The listing builds one solid part. Answer for the finished solid, in the listing's coordinates (mm). A direction names the side the tool comes from. Coordinates: 2 decimals unless noted, no trailing zeros. Order: outer loops, then holes, each group sorted by start corner. A loop starts at its lowest first (then second) coordinate and runs counter-clockwise, first axis right, second up.
from build123d import *

# Parameters (mm, degrees)
SKETCH_2_W          = 56
SKETCH_2_H          = 46.15
SKETCH_2_R          = 11
EXTRUDE_1_DEPTH     = 20
SKETCH_3_R          = 2.5
CUT_EXTRUDE_1_DEPTH = 58.565810165
SKETCH_4_W          = 3
SKETCH_4_H          = 25
CUT_EXTRUDE_2_DEPTH = 44.218312091
CHAMFER_1_SIZE      = 8
FILLET_1_R          = 1
FILLET_2_R          = 2


with BuildPart() as part:
    # 스케치2 → 보스-돌출1 (new body)
    with BuildSketch(Plane(origin=(0, 0, 0), x_dir=(0, 0, -1), z_dir=(1, 0, 0))):
        with Locations((0, -3.075)):
            Rectangle(SKETCH_2_W, SKETCH_2_H)
        Circle(SKETCH_2_R, mode=Mode.SUBTRACT)
    extrude(amount=EXTRUDE_1_DEPTH)

    # 스케치3 → 컷-돌출1 (cut, through all)
    with BuildSketch(Plane(origin=(0, 20, 0), x_dir=(1, 0, 0), z_dir=(0, 1, 0))):
        with Locations(Location((10, 20, 0), (0, 0, 270))):
            Circle(SKETCH_3_R)
        with Locations(Location((10, -20, 0), (0, 0, 90))):
            Circle(SKETCH_3_R)
    extrude(amount=-CUT_EXTRUDE_1_DEPTH, mode=Mode.SUBTRACT)

    # 스케치4 → 컷-돌출2 (cut, through all)
    with BuildSketch(Plane(origin=(20, 0, 0), x_dir=(0, 0, -1), z_dir=(1, 0, 0))):
        with Locations((-20, -3.075)):
            Rectangle(SKETCH_4_W, SKETCH_4_H)
        with Locations((20, -3.075)):
            Rectangle(SKETCH_4_W, SKETCH_4_H)
    extrude(amount=-CUT_EXTRUDE_2_DEPTH, mode=Mode.SUBTRACT)

    # 모따기1
    # the kernel refuses this chamfer: 8 mm, written as the material it takes off along each edge
    with BuildSketch(Plane(origin=(-20.573463904, 20, 28), x_dir=(0, -0.9996219169112968, 0.027495876610586494), z_dir=(1, 0, 0))) as chamfer_1_piece_1:
        Polygon((CHAMFER_1_SIZE * 0.999621916911, CHAMFER_1_SIZE * 0.0274958766106), (-CHAMFER_1_SIZE * 0.0274958766106, CHAMFER_1_SIZE * 0.999621916911), (0, 0), align=None)
    extrude(amount=61.146927807, mode=Mode.SUBTRACT)
    with BuildSketch(Plane(origin=(-20.573463904, 20, -28), x_dir=(0, -0.9996219169112968, -0.027495876610586494), z_dir=(1, 0, 0))) as chamfer_1_piece_2:
        Polygon((CHAMFER_1_SIZE * 0.999621916911, -CHAMFER_1_SIZE * 0.0274958766106), (-CHAMFER_1_SIZE * 0.0274958766106, -CHAMFER_1_SIZE * 0.999621916911), (0, 0), align=None)
    extrude(amount=61.146927807, mode=Mode.SUBTRACT)

    # 필렛1
    fillet_1_edges = [part.edges().sort_by_distance(p)[0] for p in [
        (12.5, 9.425, -20),
        (12, -3.075, -18.5),
        (12.5, -15.575, -20),
        (12, -3.075, -21.5),
        (7.5, 9.425, -20),
        (8, -3.075, -18.5),
        (7.5, -15.575, -20),
        (8, -3.075, -21.5),
        (12.5, -15.575, 20),
        (12, -3.075, 18.5),
        (12.5, 9.425, 20),
        (12, -3.075, 21.5),
        (7.5, -15.575, 20),
        (8, -3.075, 18.5),
        (7.5, 9.425, 20),
        (8, -3.075, 21.5),
    ]]
    fillet(fillet_1_edges, radius=FILLET_1_R)

    # 필렛2
    fillet_2_edges = [part.edges().sort_by_distance(p)[0] for p in [
        (0, -3.075, 21.5),
        (0, 9.425, 20),
        (0, -3.075, 18.5),
        (0, -15.575, 20),
        (20, -3.075, 21.5),
        (20, -15.575, 20),
        (20, -3.075, 18.5),
        (20, 9.425, 20),
        (0, -3.075, -21.5),
        (0, -15.575, -20),
        (0, -3.075, -18.5),
        (0, 9.425, -20),
        (20, -3.075, -21.5),
        (20, 9.425, -20),
        (20, -3.075, -18.5),
        (20, -15.575, -20),
    ]]
    fillet(fillet_2_edges, radius=FILLET_2_R)


solid = part.part
(1) Find section A-A on x = 10. Determine the outline of the cut face in (y, z).
(2) The mould has two halves that part along Z. Classify faces 1 (the flat face through (10, 16, 24)), 2 (the cylindrical face through (19.651, -16.446, 19.951)), 3 (the flat face through (10, -7, -28)): pulls with the +Z half, pulls with the -Z half, needs draft (parallel to the pull), parting line crosses it, or undercut.
(3) Given pin 1 Ø1.5 at (x, z) = (16.5, -21) entering from +Y, flat-ended and moving along its own axis, determine where the tip first touches the part or whether it passes through.
(4) Find section D-D on x = 16.5. Determine the outline of the cut face in (y, z) (3 decimals), then the cut area to 3 significant figures.
(5) Find section C-C on y = 13. Determine the outline of the cut face in (x, z), then the cut area to 3 significant figures.
(6) Find section B-B on z = 0. Determine the outline of the cut face in (x, y).
(7) A tool of negligible diameter and unlimited length cuts with its end or side. For faces 4 (the cylindrical face through (19.43, -2.87, -22.1)), 5 (the cylindrical face through (0.57, -2.87, 22.1)), 6 (the flat face through (5, -3, 21.5)), from which of +Z, -Z, +X, -X, +Y, -Y can it reach the whole face along a straight path? Write none if from no direction.
(8) Find the intervals of material crossed by probe 1 along Z at (x, y) = (1.75, -14); probe 2 along Z at (x, y) = (10, -10); probe 3 along Z at (x, y) = (9, -24), in increasing order.
Resolved:
1. outline: (-26.15, -28) - (12, -28) - (17.5, -22.5) - (-26.15, -22.5) - close; (-26.15, -17.5) - (20, -17.5) - (20, 17.5) - (-26.15, 17.5) - close; (-26.15, 22.5) - (17.5, 22.5) - (12, 28) - (-26.15, 28) - close; hole circle Ø22 at (0, 0)
2. face 1: pulls with the +Z half
2. face 2: undercut
2. face 3: pulls with the -Z half
3. pin 1: stops at y = 19.75
4. outline: (-26.15, -28) - (12, -28) - (20, -20) - (20, 20) - (12, 28) - (-26.15, 28) - close; hole (-15.575, -21.5) - (9.425, -21.5) - (9.425, -18.5) - (-15.575, -18.5) - close; hole (-15.575, 18.5) - (9.425, 18.5) - (9.425, 21.5) - (-15.575, 21.5) - close; hole circle Ø22 at (0, 0)
4. area: 1,990 mm2
5. outline: (0, -27) - (20, -27) - (20, 27) - (0, 27) - close; hole circle Ø5 at (10, -20); hole circle Ø5 at (10, 20)
5. area: 1,040 mm2
6. outline: (0, -26.15) - (20, -26.15) - (20, -11) - (0, -11) - close; (0, 11) - (20, 11) - (20, 20) - (0, 20) - close
7. face 4: +X
7. face 5: -X
7. face 6: +X, -X
8. probe 1: z = -28 to -21.52, -18.48 to 18.48, 21.52 to 28
8. probe 2: z = -28 to -22.5, -17.5 to -4.58, 4.58 to 17.5, 22.5 to 28
8. probe 3: z = -28 to -22.29, -17.71 to 17.71, 22.29 to 28
